Source: CAD feature listing. Evaluate the final solid. Frame: model axes, mm. Face numbers are marked on the shaded views. A direction names the side the tool comes from. Coordinates: 2 decimals unless noted, no trailing zeros. Loops run counter-clockwise (first coordinate to the right, second up) from the corner with the lowest first, then second, coordinate; pieces in that order, holes last.
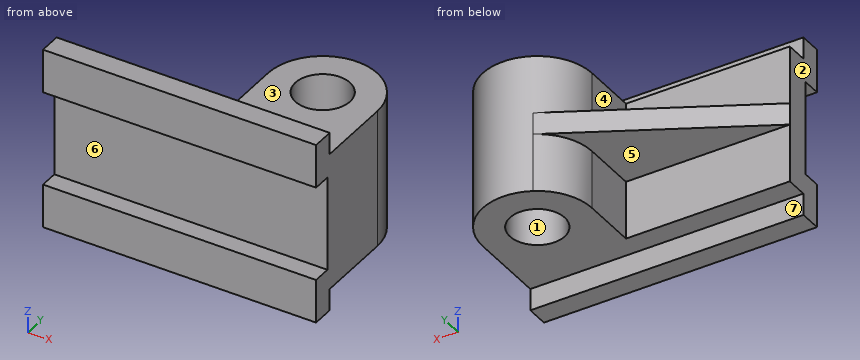
```python
from build123d import *

# Parameters (mm, degrees)
SKETCH2_W           = 90
SKETCH2_H           = 24
BOSS_EXTRUDE1_DEPTH = 76
SKETCH3_W           = 150
SKETCH3_H           = 12
BOSS_EXTRUDE2_DEPTH = 12
SKETCH4_W           = 150
SKETCH4_H           = 12
BOSS_EXTRUDE3_DEPTH = 12
SKETCH5_W           = 150
SKETCH5_H           = 52
CUT_EXTRUDE1_DEPTH  = 10
BOSS_EXTRUDE6_DEPTH = 44
CUT_EXTRUDE2_DEPTH  = 32


with BuildPart() as part:
    # Sketch2 → Boss-Extrude1 (new body)
    with BuildSketch(Plane.XY):
        with BuildLine():
            Line((30, -54), (30, 0))
            ThreePointArc((30, 0), (0, -30), (-30, 0))
            Line((-30, 0), (-30, -30))
            Line((-30, -30), (-30, -54))
            Line((-30, -54), (30, -54))
        make_face()
        with Locations((-75, -42)):
            Rectangle(SKETCH2_W, SKETCH2_H)
        with BuildLine():
            ThreePointArc((-15, 0), (0, 15), (15, 0))
            Line((15, 0), (30, 0))
            ThreePointArc((30, 0), (0, 30), (-30, 0))
            Line((-30, 0), (-15, 0))
        make_face()
        with BuildLine():
            Line((30, 0), (15, 0))
            ThreePointArc((15, 0), (0, -15), (-15, 0))
            Line((-15, 0), (-30, 0))
            ThreePointArc((-30, 0), (0, -30), (30, 0))
        make_face()
    extrude(amount=BOSS_EXTRUDE1_DEPTH)

    # Sketch3 → Boss-Extrude2 (add)
    with BuildSketch(Plane.XY.offset(76)):
        with Locations((-45, -48)):
            Rectangle(SKETCH3_W, SKETCH3_H)
    extrude(amount=BOSS_EXTRUDE2_DEPTH)

    # Sketch4 → Boss-Extrude3 (add)
    with BuildSketch(Plane(origin=(0, 0, 0), x_dir=(-1, 0, 0), z_dir=(0, 0, -1))):
        with Locations((45, -48)):
            Rectangle(SKETCH4_W, SKETCH4_H)
    extrude(amount=BOSS_EXTRUDE3_DEPTH)

    # Sketch5 → Cut-Extrude1 (cut)
    with BuildSketch(Plane(origin=(0, -54, 0), x_dir=(-1, 0, 0), z_dir=(0, -1, 0))):
        with Locations((45, -38)):
            Rectangle(SKETCH5_W, SKETCH5_H)
    extrude(amount=-CUT_EXTRUDE1_DEPTH, mode=Mode.SUBTRACT)

    # Sketch11 → Boss-Extrude6 (add)
    with BuildSketch(Plane.XY):
        with BuildLine():
            Line((-14.117647059, 26.470588235), (-120, -30))
            Line((-120, -30), (-30, -30))
            Line((-30, -30), (-30, 0))
            ThreePointArc((-30, 0), (-25.724787771, 15.434872663), (-14.117647059, 26.470588235))
        make_face()
    extrude(amount=BOSS_EXTRUDE6_DEPTH)

    # Sketch13 → Cut-Extrude2 (cut)
    with BuildSketch(Plane.XY):
        with BuildLine():
            Line((-30, -30), (-30, 0))
            ThreePointArc((-30, 0), (-25.724787771, 15.434872663), (-14.117647059, 26.470588235))
            Line((-14.117647059, 26.470588235), (-120, -30))
            Line((-120, -30), (-30, -30))
        make_face()
    extrude(amount=CUT_EXTRUDE2_DEPTH, mode=Mode.SUBTRACT)


solid = part.part
```
Q1. Section query B-B on y = 13. Return the cut outline in (x, z) (3 decimals).
Q2. Section query C-C on x = -67.5. Return the cut outline in (y, z), then the cut area to 3 significant figures.
Q3. Material intervals for line 1 along Z through (x, y) = (-22.5, -47.5); line 2 along Y through (x, z) = (0, 21.5); line 3 along Y through (x, z) = (-81, 82), sorted ascending.
Q4. Draft query along X for the marked faces 1, 2 and 3. Return one class per face: released by +X, released by -X, zero draft, split by the parting line, or undercut.
Q5. Section query D-D on y = -27.5. Return the cut outline in (x, z).
Q6. Section query A-A on x = 0. Return the cut outline in (y, z).
Q7. First-contact query: pin 1 Ø10 at (x, z) = (-79.5, 35) entering from -Y; pin 2 Ø5 at (x, z) = (-61, 50) entering from +Y; pin 3 Ø2 at (x, z) = (-4, 51.5) entering from +Y. Flat tips, straight axial feed; report the tip coordinate or a pass-through.
Q8. Reachability of the marked faces 4, 5, 6 and 7 from +Z, -Z, +X, -X, +Y, -Y: full face, straight path, thin tool, end or side. Return the list, or none.
Resolved:
1. outline: (-39.375, 32) - (-27.037, 32) - (-27.037, 0) - (-7.483, 0) - (-7.483, 76) - (-27.037, 76) - (-27.037, 44) - (-39.375, 44) - close; (7.483, 0) - (27.037, 0) - (27.037, 76) - (7.483, 76) - close
2. outline: (-54, -12) - (-42, -12) - (-42, 0) - (-30, 0) - (-30, 32) - (-2, 32) - (-2, 44) - (-30, 44) - (-30, 76) - (-42, 76) - (-42, 88) - (-54, 88) - (-54, 64) - (-44, 64) - (-44, 12) - (-54, 12) - close
2. area: 1,930 mm2
3. line 1: z = -12 to 12, 64 to 88
3. line 2: y = -44 to -15, 15 to 30
3. line 3: y = -54 to -42
4. face 1: undercut
4. face 2: released by -X
4. face 3: zero draft
5. outline: (-115.31, 32) - (-30, 32) - (-30, 0) - (30, 0) - (30, 76) - (-30, 76) - (-30, 44) - (-115.31, 44) - close
6. outline: (-54, -12) - (-42, -12) - (-42, 0) - (-15, 0) - (-15, 76) - (-42, 76) - (-42, 88) - (-54, 88) - (-54, 64) - (-44, 64) - (-44, 12) - (-54, 12) - close; (15, 0) - (30, 0) - (30, 76) - (15, 76) - close
7. pin 1: stops at y = -44
7. pin 2: stops at y = -30
7. pin 3: stops at y = 29.85
8. face 4: +Z, -X, +Y
8. face 5: -Z, -X, +Y
8. face 6: +X, -X, -Y
8. face 7: -Z, +X, -X, +Y
